Source: CAD feature listing. Evaluate the final solid. Frame: model axes, mm. Face numbers are marked on the shaded views. Give positions to 0.01 mm unless a question says otherwise; leave off trailing zeros. Write each loop counter-clockwise with the first axis right and the second up, starting at its lowest first coordinate (ties: lowest second). Pieces come first, ordered by that corner, then holes. Notation, with made-up numbers: (-7, -17.75) - (18, -17.75) arc R27 ccw to (18, 10.25) - close; hole circle Ø6 at (-14.75, 38). An arc over 180 degrees is marked (long way). One line per question, with ' | ' between items. Start each with the question number.
(1) Section C-C, the plane z = 3.5. Return loops of the section in (x, y), plus the area to 3 significant figures.
(2) Ray query, line 1 (X direction, y = 27.85, z = 0.5); line 2 (Y direction, x = 62.1, z = 3.75); line 3 (X direction, y = 27.1, z = 0.65). Return the intervals inside material, ascending. Write a range as [from, to].
(3) Section A-A, the plane x = 62.1. Return loops of the section in (y, z), plus the area to 3 significant figures.
(4) Draft query along Y for the marked faces 1, 2 and 3. Return one class per face: +Y half, -Y half, draft (parallel to the pull), parting line (faces both ways), or undercut.
(5) Section B-B, the plane y = 27.9. Return loops of the section in (x, z).
```python
from build123d import *

# Parameters (mm, degrees)
CYLINDER002002001001001001001001006_R     = 1.35
CYLINDER002002001001001001001001006_DEPTH = 5
BOX005_W                                  = 5
BOX005_H                                  = 5
BOX005_DEPTH                              = 5


with BuildPart() as cylinder002002001001001001001001006:
    # Cylinder002002001001001001001001006 → Cylinder002002001001001001001001006 (new body)
    with BuildSketch(Plane(origin=(62.1, 27.9, 0), x_dir=(1, 0, 0), z_dir=(0, 0, 1))):
        Circle(CYLINDER002002001001001001001001006_R)
    extrude(amount=CYLINDER002002001001001001001001006_DEPTH)


with BuildPart() as cut013003020:
    # Box005 → Box005 (new body)
    with BuildSketch(Plane(origin=(59.6, 25.4, 0), x_dir=(1, 0, 0), z_dir=(0, 0, 1))):
        with Locations((2.5, 2.5)):
            Rectangle(BOX005_W, BOX005_H)
    extrude(amount=BOX005_DEPTH)

    # Cut013003020: cut Cylinder002002001001001001001001006
    add(cylinder002002001001001001001001006.part, mode=Mode.SUBTRACT)


solid = cut013003020.part
```
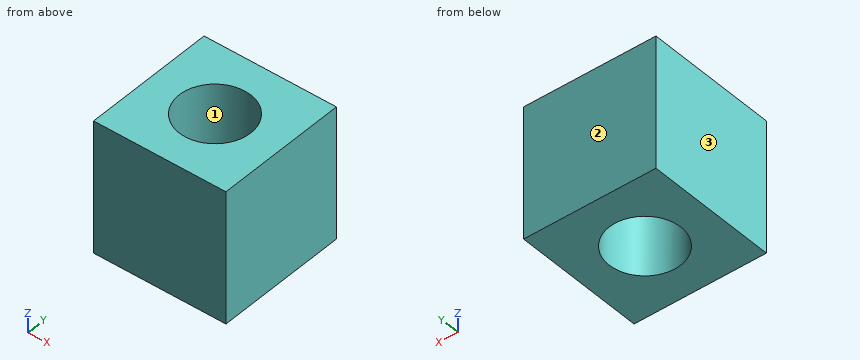
Check sheet entries:
1) outline: (59.6, 25.4) - (64.6, 25.4) - (64.6, 30.4) - (59.6, 30.4) - close; hole circle Ø2.7 at (62.1, 27.9) | area: 19.3 mm²
2) line 1: [59.6, 60.75], [63.45, 64.6] | line 2: [25.4, 26.55], [29.25, 30.4] | line 3: [59.6, 61.01], [63.19, 64.6]
3) outline: (25.4, 0) - (26.55, 0) - (26.55, 5) - (25.4, 5) - close; (29.25, 0) - (30.4, 0) - (30.4, 5) - (29.25, 5) - close | area: 11.5 mm²
4) face 1: undercut | face 2: +Y half | face 3: draft
5) outline: (59.6, 0) - (60.75, 0) - (60.75, 5) - (59.6, 5) - close; (63.45, 0) - (64.6, 0) - (64.6, 5) - (63.45, 5) - close
